For this review, use the dimensioned drawing (mm, ordinates from the lowest corner) and the shaded views. A direction names the side the tool comes from. Coordinates: 2 decimals unless noted, no trailing zeros. Loops run counter-clockwise (first coordinate to the right, second up) from the corner with the lowest first, then second, coordinate; pieces in that order, holes last.
1. Take a section at B-B, the plane y = 7.5. State the section outline as (x, z) points, then the cut area to 3 significant figures.
2. To check wall thickness, follow probe 1 along Z at (x, y) = (15.5, 1); probe 2 along X at (y, z) = (18.25, 5.5); probe 3 along Z at (x, y) = (1.25, 18.25). State the ranges of each line that lie inside material, in increasing order.
3. Take a section at C-C, the plane x = 16.25. State the section outline as (y, z) points, then the cut area to 3 significant figures.
4. Mouldability with a two-part tool opening along Z and no side actions: class the marked faces 1, 2 and 3 as pulls with the +Z half, pulls with the -Z half, needs draft (parallel to the pull), parting line crosses it, or undercut.
5. Take a section at A-A, the plane z = 29.5. State the section outline as (x, y) points.
6. Machinability: for the marked faces 4 and 5, which of the approach directions +Z, -Z, +X, -X, +Y, -Y give a long, thin tool a straight path to every point of the face, cutting with its end or side? Answer none if there is none.
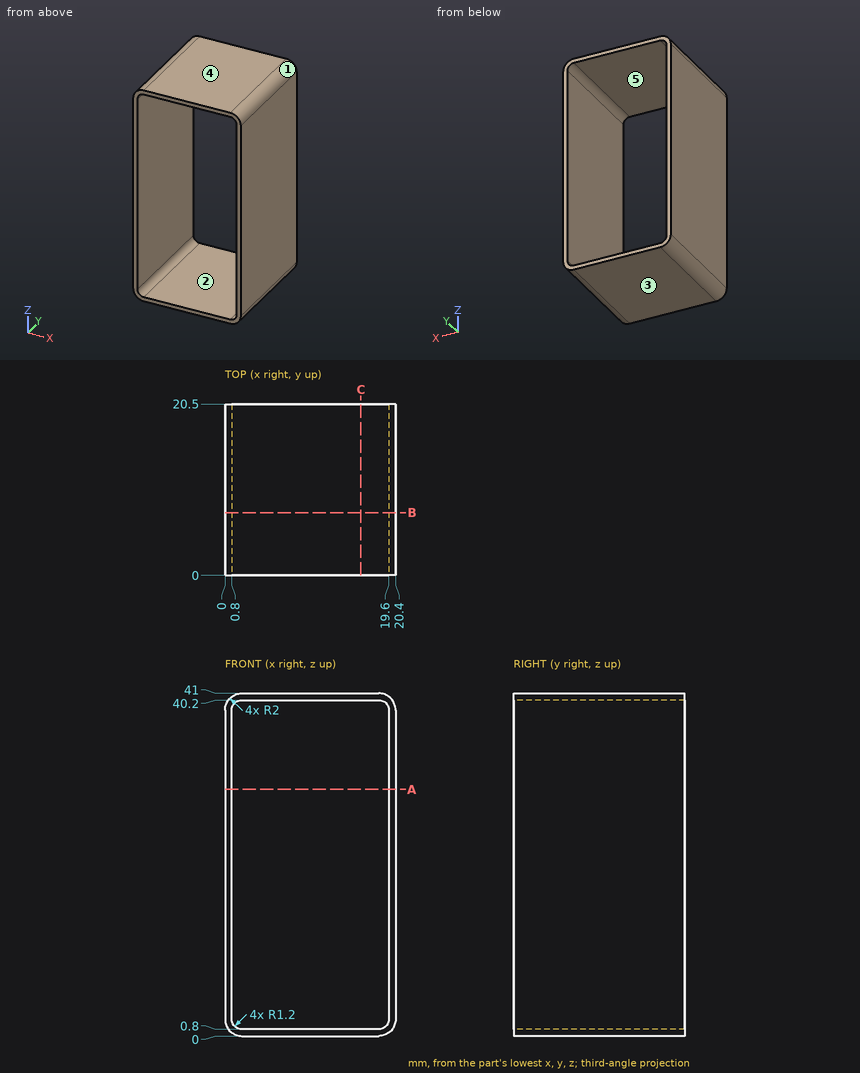
Results list:
1. outline: (0, 2) arc R2 ccw to (2, 0) - (18.4, 0) arc R2 ccw to (20.4, 2) - (20.4, 39) arc R2 ccw to (18.4, 41) - (2, 41) arc R2 ccw to (0, 39) - close; hole (0.8, 2) arc R1.2 ccw to (2, 0.8) - (18.4, 0.8) arc R1.2 ccw to (19.6, 2) - (19.6, 39) arc R1.2 ccw to (18.4, 40.2) - (2, 40.2) arc R1.2 ccw to (0.8, 39) - close
1. area: 93.5 mm2
2. probe 1: z = 0 to 0.8, 40.2 to 41
2. probe 2: x = 0 to 0.8, 19.6 to 20.4
2. probe 3: z = 0.15 to 1.06, 39.94 to 40.85
3. outline: (0, 0) - (20.5, 0) - (20.5, 0.8) - (0, 0.8) - close; (0, 40.2) - (20.5, 40.2) - (20.5, 41) - (0, 41) - close
3. area: 32.8 mm2
4. face 1: pulls with the +Z half
4. face 2: undercut
4. face 3: pulls with the -Z half
5. outline: (0, 0) - (0.8, 0) - (0.8, 20.5) - (0, 20.5) - close; (19.6, 0) - (20.4, 0) - (20.4, 20.5) - (19.6, 20.5) - close
6. face 4: +Z, +X, -X, +Y, -Y
6. face 5: +Y, -Y
